Read the model definition and answer for the solid it produces. Units are mm, in the model's axes. Give positions to 0.01 mm unless a question says otherwise; leave off trailing zeros. Order: outer loops, then holes, each group sorted by start corner. A loop starts at its lowest first (then second) coordinate and runs counter-clockwise, first axis right, second up.
Item 1: A cutting plane is placed at C-C (y = -9). Write down the section's boundary in (x, z), plus the area to 3 significant figures.
Item 2: A cutting plane is placed at B-B (y = 12.5). Write down the section's boundary in (x, z).
Item 3: Find the intervals of material crossed by line 1 along X through (y, z) = (16, 4.75); line 2 along X through (y, z) = (28.5, 7.25), in increasing order.
Item 4: A cutting plane is placed at A-A (z = 1.5). Write down the section's boundary in (x, y).
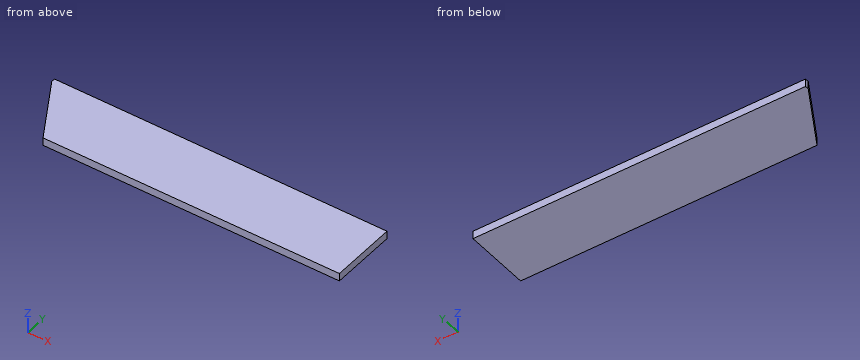
Autodesk Inventor part; units mm, degrees
ref_plane "YZ Plane" through (0, 0, 0) normal (1, 0, 0) x (0, 1, 0)
ref_plane "XZ Plane" through (0, 0, 0) normal (0, 1, 0) x (-1, 0, 0)
ref_plane "XY Plane" through (0, 0, 0) normal (0, 0, 1) x (1, 0, 0)
sketch "Sketch1" plane through (0, 0, 0) normal (0, 0, 1) x (1, 0, 0)
  line L0 (0, -42.5) -> (426, -42.5)
  line L1 (426, -42.5) -> (426, 42.5)
  line L2 (426, 42.5) -> (0, 42.5)
  line L3 (0, 42.5) -> (0, -42.5)
  line L4 (0, 37.5) -> (46.188, -42.5)
  point P0 (0, 0)
  point P1 (0, 50.9494)
  point P2 (0, 42.7975)
  point P3 (0, 0)
  dimension "d17" = 85
  dimension "d18" = 426
  dimension "d19" = 60
  dimension "d20" = 5
extrude "Plate1" add sketch "Sketch1" along normal blind 10 contours L4 L3 L2 L1 L0
equation "\"d16\" = Thickness"
equation "\"BendReliefDepth\" = 0.5 * Thickness"
properties part number "NVPH-346 feeder hose 3"
Response values:
1. outline: (26.85, 0) - (426, 0) - (426, 10) - (26.85, 10) - close
1. area: 3,990 mm2
2. outline: (14.43, 0) - (426, 0) - (426, 10) - (14.43, 10) - close
3. line 1: x = 12.41 to 426
3. line 2: x = 5.2 to 426
4. outline: (0, 37.5) - (46.19, -42.5) - (426, -42.5) - (426, 42.5) - (0, 42.5) - close
